Here's how the part is built. I have some questions about the finished solid (model axes, mm). A direction names the side the tool comes from. Give positions to 0.01 mm unless a question says otherwise; leave off trailing zeros. Write each loop counter-clockwise with the first axis right and the second up, starting at its lowest first coordinate (ties: lowest second). Pieces come first, ordered by that corner, then holes. Notation, with made-up numbers: (81, -23.5) -> (124, -23.5) arc R16 cw to (124, -17.5) -> close; hole circle Ø5 at (-25.5, -16). An arc over 180 degrees is marked (long way). Return JSON: item names as keys, results as strings.
Autodesk Inventor part; units mm, degrees
ref_plane "Work Plane1" through (-49.3077, -59.6436, 136.7512) normal (-0.0070087, 0.0889934, -0.9960076) x (-0.7423447, -0.6678024, -0.0544445)
ref_plane "YZ Plane" through (0, 0, 0) normal (1, 0, 0) x (0, 1, 0)
ref_plane "XZ Plane" through (0, 0, 0) normal (0, 1, 0) x (-1, 0, 0)
ref_plane "Work Plane1" through (-49.3077, -59.6436, 136.7512) normal (-0.0070087, 0.0889934, -0.9960076) x (-0.7423447, -0.6678024, -0.0544445)
sketch "Sketch1" plane through (-49.3077, -59.6436, 136.7512) normal (-0.0070087, 0.0889934, -0.9960076) x (-0.7423447, -0.6678024, -0.0544445)
  arc A0 (12.185, 6.495) -> (-12.185, 6.495) centre (0, 6.495) ccw
  arc A1 (12.185, 6.495) -> (-12.185, 6.495) centre (0, 6.495) ccw
  line L0 (-12.185, -6.495) -> (-12.185, 6.495)
  arc A2 (-12.185, -6.495) -> (12.185, -6.495) centre (0, -6.495) ccw
  arc A3 (-12.185, -6.495) -> (12.185, -6.495) centre (0, -6.495) ccw
  line L1 (12.185, 6.495) -> (12.185, -6.495)
  line L2 (-10.685, -6.495) -> (-10.685, 6.005)
  arc A4 (10.685, 6.495) -> (-10.685, 6.495) centre (0, 6.495) ccw
  arc A5 (-10.685, -6.495) -> (10.685, -6.495) centre (0, -6.495) ccw
  line L3 (10.685, 6.495) -> (10.685, -6.005)
  point P0 (-68.9881, 1.367)
  point P1 (10.685, 6.495)
  point P2 (10.5, -6.25)
  point P3 (-10.685, -6.495)
  point P4 (-10.5, 6.25)
  dimension "d0" = 1.5
  dimension "d1" = 1.5
  dimension "d2" = 1.5
  dimension "d3" = 1.5
extrude "Extrusion1" add sketch "Sketch1" along normal blind 50
sketch "Sketch2" plane through (-49.6582, -55.1939, 86.9509) normal (-0.0070087, 0.0889934, -0.9960076) x (-0.7423447, -0.6678024, -0.0544445)
  arc A0 (12.185, 6.495) -> (-12.185, 6.495) centre (0, 6.495) ccw
  line L0 (12.185, -6.495) -> (12.185, 6.495)
  arc A1 (-12.185, -6.495) -> (12.185, -6.495) centre (0, -6.495) ccw
  line L1 (-12.185, 6.495) -> (-12.185, -6.495)
  point P0 (-68.9881, 1.367)
extrude "Extrusion2" add sketch "Sketch2" along normal blind 2.5
sketch "Sketch3" plane through (-49.6757, -54.9714, 84.4608) normal (-0.0070087, 0.0889934, -0.9960076) x (-0.7423447, -0.6678024, -0.0544445)
  line L0 (-38, 40) -> (38, 40)
  line L1 (40, 38) -> (40, -38)
  line L2 (38, -40) -> (-38, -40)
  line L3 (-40, -38) -> (-40, 38)
  arc A0 (12.185, 6.495) -> (-12.185, 6.495) centre (0, 6.495) ccw
  line L4 (0, 40) -> (0, 18.68)
  arc A1 (-12.185, -6.495) -> (12.185, -6.495) centre (0, -6.495) ccw
  line L5 (0, -18.68) -> (0, -40)
  line L6 (-12.185, 6.495) -> (-12.185, -6.495)
  line L7 (-12.185, 0) -> (-40, 0)
  line L8 (12.185, -6.495) -> (12.185, 6.495)
  line L9 (12.185, 0) -> (40, 0)
  arc A2 (-38, 40) -> (-40, 38) centre (-38, 38) ccw
  arc A3 (40, 38) -> (38, 40) centre (38, 38) ccw
  arc A4 (-40, -38) -> (-38, -40) centre (-38, -38) ccw
  arc A5 (38, -40) -> (40, -38) centre (38, -38) ccw
  point P0 (-68.9881, 1.367)
  point P1 (-40, 40)
  point P2 (40, -40)
  point P3 (-40, -40)
  dimension "d8" = 80
  dimension "d9" = 80
  dimension "d11" = 2
  dimension "d12" = 2
  dimension "d13" = 2
  dimension "d14" = 2
extrude "Extrusion3" add sketch "Sketch3" along normal blind 2.5
chamfer "Chamfer1" distance 5 angle 45 4 edges at (-58.7212, -63.1086, 83.7974) (-62.1909, -41.1669, 85.7823) (-40.6302, -46.8343, 85.1242) (-37.1604, -68.7759, 83.1393)
properties part number "Staging_area"
1. If I drill on line 1 (Z direction, x = -15.5, y = -56); line 2 (Z direction, x = -33, y = -55.5); line 3 (X direction, y = -50, z = 135), over which ranges is the centre line in solid material (lowest first)? Write a range as [from, to].
Taken from the geometry:
{"line 1": "z = [81.62, 84.13]", "line 2": "z = [81.79, 88.35]", "line 3": "x = [-64.95, -41.44]"}
2. Which directions (+Z, -Z, +X, -X, +Y, -Y) give clear straight access to the entire face, cutting with the end or side of a thin tool? Please do faces 5 (the face through (-38.79, -45.29, 87.72)), 6 (the face through (-36.72, -69.24, 87.8)), 7 (the face through (-76.09, -24.95, 86.09)), 8 (the face through (-58.58, -65.63, 112.77)).
Taken from the geometry:
{"face 5": "+Z, +X", "face 6": "none", "face 7": "+Z, -X, +Y", "face 8": "-X, -Y"}
3. Suppose I cut it at A-A, the plane x = -77. List the corners of the cut face in (y, z) for me.
Taken from the geometry:
{"outline": "(-84.3, 82.03) -> (-84.09, 79.54) -> (-25.65, 84.76) -> (-25.88, 87.25) -> close"}
4. Suppose I cut it at B-B, the plane x = -24.5. List the corners of the cut face in (y, z) for me, and give its area (3 significant figures).
Taken from the geometry:
{"outline": "(-85.99, 81.51) -> (-85.75, 79.02) -> (-23.07, 84.62) -> (-23.28, 87.12) -> close", "area": "157 mm²"}
5. For pin 1 Ø2 at (x, z) = (-66, 103.5) entering from +Y; pin 2 Ø8 at (y, z) = (-73, 94) entering from -X; pin 3 Ø4 at (y, z) = (-55, 127) entering from +X; pin 4 Ø3 at (x, y) = (-71.5, -94.5) entering from -Z, each with a flat end and sliding along its axis, tell me the tip position at first contact or that it passes through.
Taken from the geometry:
{"pin 1": "stops at y = -46.78", "pin 2": "stops at x = -54.18", "pin 3": "stops at x = -34.77", "pin 4": "passes through"}
6. If we mould it in two halves opening along Z, with no side actions, what happens to faces 1 (the face through (-23.3, -84.8, 80.4)), 2 (the face through (5.98, -57.69, 82.59)), 3 (the face through (-61.79, -43.58, 114.76)), 4 (the face through (-40.365, -49.49, 114.084))? For each: released by +Z, released by -Z, zero draft, split by the parting line, or undercut.
Taken from the geometry:
{"face 1": "released by -Z", "face 2": "split by the parting line", "face 3": "undercut", "face 4": "released by +Z"}
